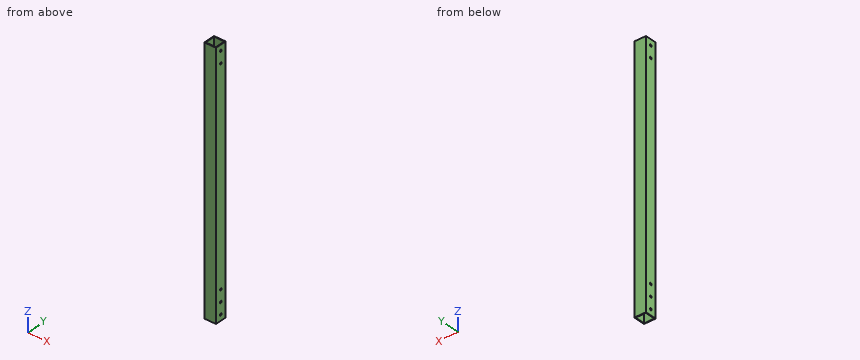
Autodesk Inventor part; units mm, degrees
ref_plane "YZ Plane" through (0, 0, 0) normal (1, 0, 0) x (0, 1, 0)
ref_plane "XZ Plane" through (0, 0, 0) normal (0, 1, 0) x (-1, 0, 0)
ref_plane "XY Plane" through (0, 0, 0) normal (0, 0, 1) x (1, 0, 0)
sketch "Sketch1" plane through (0, 0, 0) normal (0, 0, 1) x (1, 0, 0)
  line L0 (0, 0) -> (25.4, 0)
  line L1 (25.4, 0) -> (25.4, 25.4)
  line L2 (25.4, 25.4) -> (0, 25.4)
  line L3 (0, 25.4) -> (0, 0)
  dimension "d0" = 25.4
  dimension "d1" = 25.4
extrude "Extrusion1" add sketch "Sketch1" along normal blind 558.8
shell "Shell1" thickness 1.5875 removed faces 2 at (16.9333, 8.4667, 0) at (16.9333, 8.4667, 558.8)
sketch "Sketch2" plane through (25.4, 0, 0) normal (1, 0, 0) x (0, 0, -1)
  line L0 (-558.8, 25.4) -> (-558.8, 0)
  line L1 (0, 25.4) -> (-558.8, 25.4)
  circle A0 centre (-546.1, 12.7) radius 2.3813
  circle A1 centre (-520.7, 12.7) radius 2.3813
  dimension "d5" = 12.7
  dimension "d6" = 12.7
  dimension "d7" = 25.4
  dimension "d8" = 12.7
  dimension "d9" = 4.7625
  dimension "d10" = 4.7625
extrude "Extrusion2" cut sketch "Sketch2" against normal through all
sketch "Sketch3" plane through (25.4, 0, 0) normal (1, 0, 0) x (0, 0, -1)
  line L0 (0, 0) -> (0, 25.4)
  line L1 (0, 25.4) -> (-558.8, 25.4)
  circle A0 centre (-12.7, 12.7) radius 2.3813
  circle A1 centre (-38.1, 12.7) radius 2.3813
  circle A2 centre (-63.5, 12.7) radius 2.3813
  line L2 (-63.5, 12.7) -> (-38.1, 12.7) construction
  line L3 (-38.1, 12.7) -> (-12.7, 12.7) construction
  dimension "d13" = 12.7
  dimension "d14" = 25.4
  dimension "d15" = 12.7
  dimension "d16" = 4.7625
extrude "Extrusion3" cut sketch "Sketch3" against normal through all
properties part number "Frame_RearVerticalSupport" material "Aluminum-6061"
Input: part model. Units: mm. Frame: model coordinates. Give positions to 0.01 mm unless a question says otherwise; leave off trailing zeros. Loops run counter-clockwise (first coordinate to the right, second up) from the corner with the lowest first, then second, coordinate; pieces in that order, holes last. Notation, with made-up numbers: (66.5, 2.5) - (102.5, 2.5) arc R34 ccw to (102.5, 34.5) - close; hole circle Ø5 at (83.25, -22.5). An arc over 180 degrees is marked (long way). Use CSV: the item, a comma, the result in double quotes. Start each with the question number.
Item 1: Section A-A on x = 12.5. Return loops of the section in (y, z).
Item 2: Line query: line 1 (X direction, y = 15.25, z = 508.5); line 2 (Y direction, x = 0.7, z = 520.7). Output: solid intervals per line, ascending.
Item 3: Section B-B on z = 149. Return loops of the section in (x, y).
Ans:
1,outline,"(0, 0) - (1.59, 0) - (1.59, 558.8) - (0, 558.8) - close; (23.81, 0) - (25.4, 0) - (25.4, 558.8) - (23.81, 558.8) - close"
2,line 1,"x = 0 to 1.59, 23.81 to 25.4"
2,line 2,"y = 0 to 10.32, 15.08 to 25.4"
3,outline,"(0, 0) - (25.4, 0) - (25.4, 25.4) - (0, 25.4) - close; hole (1.59, 1.59) - (23.81, 1.59) - (23.81, 23.81) - (1.59, 23.81) - close"
